Could you check a few things on this model? Use its own coordinates, in mm. A direction names the side the tool comes from. Give positions to 0.01 mm unless a question says otherwise; leave off trailing zeros. Order: outer loops, then holes, each group sorted by start corner. A loop starts at its lowest first (then second) coordinate and runs counter-clockwise, first axis right, second up. Notation, with made-up numbers: (-29, 15) - (-14, 15) arc R15 cw to (-14, 21) - close; hole circle Ø4 at (65, 24). An arc over 180 degrees is marked (long way). Put each result on its own line as item: value.
from build123d import *

# Parameters (mm, degrees)
F0_W     = 37.5
F0_H     = 12
F1_DEPTH = 6
F2_W     = 36.5
F2_H     = 11
F3_DEPTH = 5.5
F4_SIZE  = 1


with BuildPart() as f1:
    # F0 (on Top) → F1 (new body)
    with BuildSketch(Plane.XY):
        with Locations((18.75, 6)):
            Rectangle(F0_W, F0_H)
    extrude(amount=F1_DEPTH)

    # F2 (on face) → F3 (cut)
    with BuildSketch(Plane.XY.offset(6)):
        with Locations((18.75, 6)):
            Rectangle(F2_W, F2_H)
    extrude(amount=-F3_DEPTH, mode=Mode.SUBTRACT)

    # F4
    f4_edges = [f1.edges().sort_by_distance(p)[0] for p in [
        (18.75, 11.5, 0.5),
        (18.75, 0.5, 0.5),
    ]]
    chamfer(f4_edges, length=F4_SIZE)


solid = f1.part
1) We'd pull the mould along Y, two halves only. Please class faces 3 (the flat face through (18, 6, 0.5)), 4 (the flat face through (18, 12, 3)), 5 (the flat face through (37.5, 6, 3)): pulls with the +Y half, pulls with the -Y half, needs draft (parallel to the pull), parting line crosses it, or undercut.
Filled in:
face 3: undercut
face 4: pulls with the +Y half
face 5: needs draft
2) Suppose I cut it at A-A, the plane z = 1.15. List the corners of the cut face in (x, y) for me, and give its area (4 significant figures).
Filled in:
outline: (0, 0) - (37.5, 0) - (37.5, 12) - (0, 12) - close; hole (0.5, 0.85) - (37, 0.85) - (37, 11.15) - (0.5, 11.15) - close
area: 74.05 mm^2
3) Which directions (+Z, -Z, +X, -X, +Y, -Y) give clear straight access to the entire face, cutting with the end or side of a thin tool? Please do faces 1 (the flat face through (0, 6, 3)), 2 (the flat face through (18, 11, 1)).
Filled in:
face 1: +Z, -Z, -X, +Y, -Y
face 2: +Z
4) If I drill on line 1 (Y direction, x = 20, z = 2.1); line 2 (X direction, y = 4.5, z = 4.1); line 3 (Z direction, x = 22, y = 5.75), over which ranges is the centre line in solid material (lowest first)? Write a range as [from, to].
Filled in:
line 1: y = [0, 0.5], [11.5, 12]
line 2: x = [0, 0.5], [37, 37.5]
line 3: z = [0, 0.5]
5) Suppose I cut it at B-B, the plane x = 30. List the corners of the cut face in (y, z) for me, and give its area (3 significant figures).
Filled in:
outline: (0, 0) - (12, 0) - (12, 6) - (11.5, 6) - (11.5, 1.5) - (10.5, 0.5) - (1.5, 0.5) - (0.5, 1.5) - (0.5, 6) - (0, 6) - close
area: 12.5 mm^2
6) Suppose I cut it at D-D, the plane z = 3.15. List the corners of the cut face in (x, y) for me, and give its area (3 significant figures).
Filled in:
outline: (0, 0) - (37.5, 0) - (37.5, 12) - (0, 12) - close; hole (0.5, 0.5) - (37, 0.5) - (37, 11.5) - (0.5, 11.5) - close
area: 48.5 mm^2
7) Suppose I cut it at C-C, the plane y = 10. List the corners of the cut face in (x, z) for me.
Filled in:
outline: (0, 0) - (37.5, 0) - (37.5, 6) - (37, 6) - (37, 0.5) - (0.5, 0.5) - (0.5, 6) - (0, 6) - close
